from build123d import *

# Parameters (mm, degrees)
F0_W           = 13.6
F0_H           = 11.85
F1_DEPTH       = 5.75
F2_T           = -1.25
F3_W           = 2.5
F3_H           = 1.25
F4_DEPTH       = 1
F6_W           = 5
F6_H           = 1.15
F7_DEPTH       = 1.5
F9_DEPTH       = 1.5
F10_W          = 4.3600509252
F10_H          = 4.6871736337
F11_DEPTH      = 7.801
F11_DEPTH_BACK = 7.801
F13_W          = 2.5
F13_H          = 0.625
F14_DEPTH      = 3
F15_W          = 2.5
F15_H          = 0.625
F16_DEPTH      = 3
F18_DEPTH      = 3
F19_R          = 3.75
F20_DEPTH      = 1.25
F20_DEPTH_BACK = 0.5
F21_R          = 3.75
F22_DEPTH      = 2.7
F22_DEPTH_BACK = 1
F24_DEPTH      = 0.2
F12_R          = 0.875
F25_DEPTH      = 0.4


with BuildPart() as f1:
    # F0 (on Top) → F1 (new body)
    with BuildSketch(Plane.XY):
        Rectangle(F0_W, F0_H)
    extrude(amount=F1_DEPTH)

    # F2
    f2_openings = [f1.faces().sort_by_distance(p)[0] for p in [
        (0, 0, 5.75),
    ]]
    offset(amount=F2_T, openings=f2_openings)

    # F3 (on face) → F4 (join)
    with BuildSketch(Plane.YZ.offset(6.8)):
        with Locations((-2.175, 1.875)):
            Rectangle(F3_W, F3_H)
    extrude(amount=F4_DEPTH)

    # F5: F1 across plane


with BuildPart() as f1_1:
    add(f1.part)
    add(f1.part.mirror(Plane.YZ))

    # F6 (on face) → F7 (join)
    with BuildSketch(Plane.XZ.offset(5.925)):
        with Locations((0, 3.075)):
            Rectangle(F6_W, F6_H)
    extrude(amount=F7_DEPTH)

    # F8 (on face) → F9 (join)
    with BuildSketch(Plane(origin=(0, 5.925, 0), x_dir=(-1, 0, 0), z_dir=(0, 1, 0))):
        with BuildLine():
            Line((-4.7, 2.7), (-2.75, 2.7))
            ThreePointArc((-2.75, 2.7), (-2.0782485579, 2.9782485579), (-1.8, 3.65))
            ThreePointArc((-1.8, 3.65), (-2.0782485579, 4.3217514421), (-2.75, 4.6))
            Line((-2.75, 4.6), (-4.7, 4.6))
            ThreePointArc((-4.7, 4.6), (-5.3717514421, 4.3217514421), (-5.65, 3.65))
            ThreePointArc((-5.65, 3.65), (-5.3717514421, 2.9782485579), (-4.7, 2.7))
        make_face()
    extrude(amount=F9_DEPTH)

    # F10 (on Right) → F11 (cut, two sides)
    with BuildSketch(Plane.YZ) as f11_sk:
        with Locations((-5.6050254626, 3.5935868168)):
            Rectangle(F10_W, F10_H)
    extrude(amount=-F11_DEPTH, mode=Mode.SUBTRACT)
    extrude(f11_sk.sketch, amount=F11_DEPTH_BACK, mode=Mode.SUBTRACT)

    # F13 (on face) → F14 (join)
    with BuildSketch(Plane.YZ.offset(7.8)):
        with Locations((-2.175, 1.5625)):
            Rectangle(F13_W, F13_H)
    extrude(amount=F14_DEPTH)

    # F15 (on face) → F16 (join)
    with BuildSketch(Plane(origin=(-7.8, 0, 0), x_dir=(0, -1, 0), z_dir=(-1, 0, 0))):
        with Locations((2.175, 1.5625)):
            Rectangle(F15_W, F15_H)
    extrude(amount=F16_DEPTH)

    # F17 (on face) → F18 (join)
    with BuildSketch(Plane(origin=(0, 7.425, 0), x_dir=(-1, 0, 0), z_dir=(0, 1, 0))):
        with BuildLine():
            Line((-4.7, 2.7), (-2.75, 2.7))
            ThreePointArc((-2.75, 2.7), (-2.0782485579, 2.9782485579), (-1.8, 3.65))
            Line((-1.8, 3.65), (-5.65, 3.65))
            ThreePointArc((-5.65, 3.65), (-5.3717514421, 2.9782485579), (-4.7, 2.7))
        make_face()
    extrude(amount=F18_DEPTH)

    # F19 (on face) → F20 (join, two sides)
    with BuildSketch(Plane(origin=(0, 0, 1.25), x_dir=(1, 0, 0), z_dir=(0, 0, -1))) as f20_sk:
        with Locations((-14.0194073319, 2.175)):
            Circle(F19_R)
        with Locations((14.0194073319, 2.175)):
            Circle(F19_R)
    extrude(amount=F20_DEPTH)
    extrude(f20_sk.sketch, amount=-F20_DEPTH_BACK)

    # F21 (on face) → F22 (join, two sides)
    with BuildSketch(Plane(origin=(0, 0, 2.7), x_dir=(1, 0, 0), z_dir=(0, 0, -1))) as f22_sk:
        with Locations((3.725, -13.0435097963)):
            Circle(F21_R)
    extrude(amount=F22_DEPTH)
    extrude(f22_sk.sketch, amount=-F22_DEPTH_BACK)

    # F23 (on Top) → F24 (join)
    with BuildSketch(Plane.XY):
        with BuildLine():
            Line((1.2836985293, 15.8900071403), (-16.4607088026, 0.6714973441))
            ThreePointArc((-16.4607088026, 0.6714973441), (-17.536285567, -3.4765634752), (-14.0194073319, -5.925))
            Line((-14.0194073319, -5.925), (14.0194073319, -5.925))
            ThreePointArc((14.0194073319, -5.925), (17.3316275311, -3.9333223118), (17.1255143602, -0.0739052545))
            Line((17.1255143602, -0.0739052545), (6.8311070282, 15.1446045417))
            ThreePointArc((6.8311070282, 15.1446045417), (4.2243975028, 16.7601079901), (1.2836985293, 15.8900071403))
        make_face()
    extrude(amount=F24_DEPTH)

    # F12 (on Top) → F25 (cut)
    with BuildSketch(Plane.XY):
        with Locations((0, -4.125)):
            Circle(F12_R)
        with BuildLine():
            ThreePointArc((4.3735203272, 2.1210343377), (5.4180666877, 2.3052160437), (5.2338849817, 3.3497624041))
            ThreePointArc((5.2338849817, 3.3497624041), (0, 5), (-5.2338849817, 3.3497624041))
            ThreePointArc((-5.2338849817, 3.3497624041), (-5.4180666877, 2.3052160437), (-4.3735203272, 2.1210343377))
            ThreePointArc((-4.3735203272, 2.1210343377), (0, 3.5), (4.3735203272, 2.1210343377))
        make_face()
        with BuildLine():
            ThreePointArc((2.7961851272, -0.1316337841), (3.8407314877, 0.0525479219), (3.6565497817, 1.0970942823))
            ThreePointArc((3.6565497817, 1.0970942823), (0, 2.25), (-3.6565497817, 1.0970942823))
            ThreePointArc((-3.6565497817, 1.0970942823), (-3.8407314877, 0.0525479219), (-2.7961851272, -0.1316337841))
            ThreePointArc((-2.7961851272, -0.1316337841), (0, 0.75), (2.7961851272, -0.1316337841))
        make_face()
        with BuildLine():
            ThreePointArc((1.2188499272, -2.3843019059), (2.2633962877, -2.2001201999), (2.0792145818, -1.1555738395))
            ThreePointArc((2.0792145818, -1.1555738395), (0, -0.5), (-2.0792145818, -1.1555738395))
            ThreePointArc((-2.0792145818, -1.1555738395), (-2.2633962877, -2.2001201999), (-1.2188499272, -2.3843019059))
            ThreePointArc((-1.2188499272, -2.3843019059), (0, -2), (1.2188499272, -2.3843019059))
        make_face()
    extrude(amount=F25_DEPTH, mode=Mode.SUBTRACT)


solid = f1_1.part
Design review of the part built by this model. Coordinates are the model's own, in mm. A direction names the side the tool comes from. Give positions to 0.01 mm unless a question says otherwise; leave off trailing zeros. Loops run counter-clockwise (first coordinate to the right, second up) from the corner with the lowest first, then second, coordinate; pieces in that order, holes last. Notation, with made-up numbers: M -8,38.25 L 8,38.25 A20 ccw 8,51.25 Z; hole C 50,3 d9. An arc over 180 degrees is marked long. Answer as a JSON object with one key per item and string values.
Item 1: We need section A-A (x = -9). State the section outline as (y, z) points (3 decimals).
Output values:
{"outline": "M -5.925,0 L 7.07,0 L 7.07,0.2 L -5.925,0.2 Z; M -3.425,1.25 L -0.925,1.25 L -0.925,1.875 L -3.425,1.875 Z"}
Item 2: For P1, Ø5.5, axis at x = -1.5, y = 1.5, coming from the +Z side; P2, Ø0.8, axis at x = -9, y = -2, coming from the +Z side (3 decimals); P3, Ø1.5, axis at x = 1.5, z = 3.5, coming from the +Y side, all flat-tipped, find the tip position at first contact; note any pin that passes through.
Output values:
{"P1": "stops at z = 1.25", "P2": "stops at z = 1.875", "P3": "stops at y = 16.49"}
Item 3: We need section C-C (x = 16). State the section outline as (y, z) points, and give its area (3 significant figures).
Output values:
{"outline": "M -5.36,0 L 1.59,0 L 1.59,0.2 L 1.01,0.2 L 1.01,1.75 L -5.36,1.75 Z", "area": "11.3 mm2"}
Item 4: Mouldability with a two-part tool opening along X and no side actions: class faces 4 (the face through (4, 7, 4.6)), 5 (the face through (-6.8, 1, 3)) as pulls with the +X half, pulls with the -X half, needs draft (parallel to the pull), parting line crosses it, or undercut.
Output values:
{"face 4": "needs draft", "face 5": "undercut"}
Item 5: We need section D-D (y = 10.75). State the section outline as (x, z) points, and give its area (3 significant figures).
Output values:
{"outline": "M -4.71,0 L 9.8,0 L 9.8,0.2 L 6.69,0.2 L 6.69,3.7 L 0.76,3.7 L 0.76,0.2 L -4.71,0.2 Z", "area": "23.7 mm2"}
Item 6: We need section B-B (z = 4.2). State the section outline as (x, y) points (3 decimals).
Output values:
{"outline": "M -6.8,-3.425 L -5.55,-3.425 L -5.55,4.675 L 5.55,4.675 L 5.55,-3.425 L 6.8,-3.425 L 6.8,5.925 L 5.475,5.925 L 5.475,7.425 L 1.975,7.425 L 1.975,5.925 L -6.8,5.925 Z"}
Item 7: Wall thickness on line 1 along X through (y, z) = (3.5, 2.5); line 2 along X through (y, z) = (-3, 0.9); line 3 along Z through (x, y) = (7, 7.75): over which ranges is each line inside the solid? List them lowest first.
Output values:
{"line 1": "x = -6.8 to -5.55, 5.55 to 6.8", "line 2": "x = -17.68 to -10.36, -6.8 to 6.8, 10.36 to 17.68", "line 3": "z = 0 to 0.2"}
Item 8: Machinability: for faces 1 (the face through (0.81, -4.46, 0.2)), 2 (the face through (7, -2, 2.5)), 3 (the face through (-7, -3.425, 2)), which of the approach directions +Z, -Z, +X, -X, +Y, -Y give a long, thin tool a straight path to every point of the face, cutting with its end or side? Answer none if there is none.
Output values:
{"face 1": "-Z", "face 2": "+Z, +X, -Y", "face 3": "+Z, -Y"}
